Geometry: final body of the model. Coordinates: model frame, mm. Give positions to 0.01 mm unless a question says otherwise; leave off trailing zeros. Answer in a Markdown table with one row per item. Add a question column.
1) Draft query along Z for faces 1 (the flat face through (-2.4, 0.1, 400)), 2 (the flat face through (10, 6, 197)), 3 (the flat face through (-2.4, 0.1, 0)). Return one class per face: +Z half, -Z half, draft (parallel to the pull), parting line (faces both ways), or undercut.
2) Line query: line 1 (Y direction, x = -7.5, z = 163.5); line 2 (Y direction, x = -7, z = 193.5). Output: solid intervals per line, ascending. Write a range as from..to.
3) Section query A-A (z = 105). Give the number of separate pieces and of enclosed holes in the cut face, plus the area to 3 significant figures.
Autodesk Inventor part; units mm, degrees
ref_plane "YZ Plane" through (0, 0, 0) normal (1, 0, 0) x (0, 1, 0)
ref_plane "XZ Plane" through (0, 0, 0) normal (0, 1, 0) x (-1, 0, 0)
ref_plane "XY Plane" through (0, 0, 0) normal (0, 0, 1) x (1, 0, 0)
sketch "Sketch1" plane through (0, 0, 0) normal (0, 0, 1) x (1, 0, 0)
  line L0 (0, 0) -> (12.2143, 12.2143) construction
  line L1 (0, 0) -> (10, 0) construction
  circle A0 centre (0, 0) radius 2.15
  circle A1 centre (7, 7) radius 2
  circle A2 centre (-7, 7) radius 2
  circle A3 centre (-7, -7) radius 2
  circle A4 centre (7, -7) radius 2
  line L2 (2.95, 10) -> (9.5, 10)
  line L3 (10, 9.5) -> (10, 2.95)
  line L4 (9.7, 2.65) -> (8.9, 2.65)
  line L5 (8.6, 2.95) -> (8.6, 4.2)
  line L6 (4.2, 4.4357) -> (4.2, 8.6)
  line L7 (2.65, 9.7) -> (2.65, 8.9)
  line L8 (2.95, 8.6) -> (4.2, 8.6)
  line L9 (0, 14.2934) -> (0, -14.2934) construction
  arc A5 (2.95, 10) -> (2.65, 9.7) centre (2.95, 9.7) ccw
  arc A6 (2.65, 8.9) -> (2.95, 8.6) centre (2.95, 8.9) ccw
  arc A7 (8.6, 2.95) -> (8.9, 2.65) centre (8.9, 2.95) ccw
  arc A8 (9.7, 2.65) -> (10, 2.95) centre (9.7, 2.95) ccw
  arc A9 (10, 9.5) -> (9.5, 10) centre (9.5, 9.5) ccw
  circle A10 centre (0, 7.1516) radius 5.0016 construction
  circle A11 centre (7.1516, 0) radius 5.0016 construction
  line L10 (8.6, 4.2) -> (4.4357, 4.2)
  line L11 (0, 3) -> (1.9054, 3.3)
  arc A12 (1.9054, 3.3) -> (4.2, 4.4357) centre (0, 10.0357) ccw
  line L12 (3, 0) -> (3.3, 1.9054)
  arc A13 (4.4357, 4.2) -> (3.3, 1.9054) centre (10.0357, 0) ccw
  line L13 (-3, 0) -> (-3.3, 1.9054)
  arc A14 (-3.3, 1.9054) -> (-4.4357, 4.2) centre (-10.0357, 0) ccw
  arc A15 (-4.2, 4.4357) -> (-1.9054, 3.3) centre (0, 10.0357) ccw
  line L14 (0, 3) -> (-1.9054, 3.3)
  line L15 (-4.4357, 4.2) -> (-8.6, 4.2)
  line L16 (-8.6, 2.95) -> (-8.6, 4.2)
  arc A16 (-8.9, 2.65) -> (-8.6, 2.95) centre (-8.9, 2.95) ccw
  line L17 (-9.7, 2.65) -> (-8.9, 2.65)
  arc A17 (-10, 2.95) -> (-9.7, 2.65) centre (-9.7, 2.95) ccw
  line L18 (-10, 2.95) -> (-10, 9.5)
  arc A18 (-9.5, 10) -> (-10, 9.5) centre (-9.5, 9.5) ccw
  line L19 (-9.5, 10) -> (-2.95, 10)
  line L20 (-4.2, 8.6) -> (-4.2, 4.4357)
  line L21 (-2.95, 8.6) -> (-4.2, 8.6)
  arc A19 (-2.95, 8.6) -> (-2.65, 8.9) centre (-2.95, 8.9) ccw
  line L22 (-2.65, 9.7) -> (-2.65, 8.9)
  arc A20 (-2.65, 9.7) -> (-2.95, 10) centre (-2.95, 9.7) ccw
  line L23 (0, -3) -> (-1.9054, -3.3)
  arc A21 (-1.9054, -3.3) -> (-4.2, -4.4357) centre (0, -10.0357) ccw
  arc A22 (-4.4357, -4.2) -> (-3.3, -1.9054) centre (-10.0357, 0) ccw
  line L24 (-3, 0) -> (-3.3, -1.9054)
  line L25 (-4.2, -4.4357) -> (-4.2, -8.6)
  line L26 (-2.95, -8.6) -> (-4.2, -8.6)
  arc A23 (-2.65, -8.9) -> (-2.95, -8.6) centre (-2.95, -8.9) ccw
  line L27 (-2.65, -9.7) -> (-2.65, -8.9)
  arc A24 (-2.95, -10) -> (-2.65, -9.7) centre (-2.95, -9.7) ccw
  line L28 (-2.95, -10) -> (-9.5, -10)
  arc A25 (-10, -9.5) -> (-9.5, -10) centre (-9.5, -9.5) ccw
  line L29 (-10, -9.5) -> (-10, -2.95)
  line L30 (-8.6, -4.2) -> (-4.4357, -4.2)
  line L31 (-8.6, -2.95) -> (-8.6, -4.2)
  arc A26 (-8.6, -2.95) -> (-8.9, -2.65) centre (-8.9, -2.95) ccw
  line L32 (-9.7, -2.65) -> (-8.9, -2.65)
  arc A27 (-9.7, -2.65) -> (-10, -2.95) centre (-9.7, -2.95) ccw
  line L33 (3, 0) -> (3.3, -1.9054)
  arc A28 (3.3, -1.9054) -> (4.4357, -4.2) centre (10.0357, 0) ccw
  arc A29 (4.2, -4.4357) -> (1.9054, -3.3) centre (0, -10.0357) ccw
  line L34 (0, -3) -> (1.9054, -3.3)
  line L35 (4.4357, -4.2) -> (8.6, -4.2)
  line L36 (8.6, -2.95) -> (8.6, -4.2)
  arc A30 (8.9, -2.65) -> (8.6, -2.95) centre (8.9, -2.95) ccw
  line L37 (9.7, -2.65) -> (8.9, -2.65)
  arc A31 (10, -2.95) -> (9.7, -2.65) centre (9.7, -2.95) ccw
  line L38 (10, -2.95) -> (10, -9.5)
  arc A32 (9.5, -10) -> (10, -9.5) centre (9.5, -9.5) ccw
  line L39 (9.5, -10) -> (2.95, -10)
  line L40 (4.2, -8.6) -> (4.2, -4.4357)
  line L41 (2.95, -8.6) -> (4.2, -8.6)
  arc A33 (2.95, -8.6) -> (2.65, -8.9) centre (2.95, -8.9) ccw
  line L42 (2.65, -9.7) -> (2.65, -8.9)
  arc A34 (2.65, -9.7) -> (2.95, -10) centre (2.95, -9.7) ccw
  point P0 (10, 2.65)
  point P1 (8.6, 2.65)
  point P2 (-2.65, 10)
  point P3 (-2.65, 8.6)
  point P4 (-10, -2.65)
  point P5 (-8.6, -2.65)
  point P6 (2.65, -10)
  point P7 (2.65, -8.6)
  dimension "d1" = 45
  dimension "d2" = 4.3
  dimension "d3" = 4
  dimension "d6" = 360
  dimension "d9" = 2.65
  dimension "d10" = 4.2
  dimension "d11" = 1.4
  dimension "d12" = 7
  dimension "d13" = 10
  dimension "d14" = 10
  dimension "d15" = 1.4
  dimension "d16" = 2.65
  dimension "d18" = 0.3
  dimension "d19" = 0.5
  dimension "d22" = 4.2
  dimension "d24" = 6.7
  dimension "d25" = 0.3
  dimension "d26" = 7
  dimension "d27" = 6.7
  dimension "d28" = 0.3
  dimension "d29" = 7
  dimension "d32" = 360
extrude "Extrusion1" add sketch "Sketch1" along normal blind 400
sketch "Sketch2" plane through (2.95, 10, 400) normal (0, 1, 0) x (1, 0, 0)
  line L0 (-2.95, 400) -> (-2.95, 0)
  circle A0 centre (-2.95, 6) radius 2.15
  dimension "d36" = 4.3
  dimension "d37" = 6
extrude "Extrusion2" cut sketch "Sketch2" against normal blind 10
properties part number "Aluminum_Profile_2020"
Evaluation:
| question | item | result |
|---|---|---|
| 1 | face 1 | +Z half |
| 1 | face 2 | draft |
| 1 | face 3 | -Z half |
| 2 | line 1 | -10..-8.94, -5.06..-4.2, 4.2..5.06, 8.94..10 |
| 2 | line 2 | -10..-9, -5..-4.2, 4.2..5, 9..10 |
| 3 | separate pieces | 1 |
| 3 | enclosed holes | 5 |
| 3 | area | 133 mm² |
